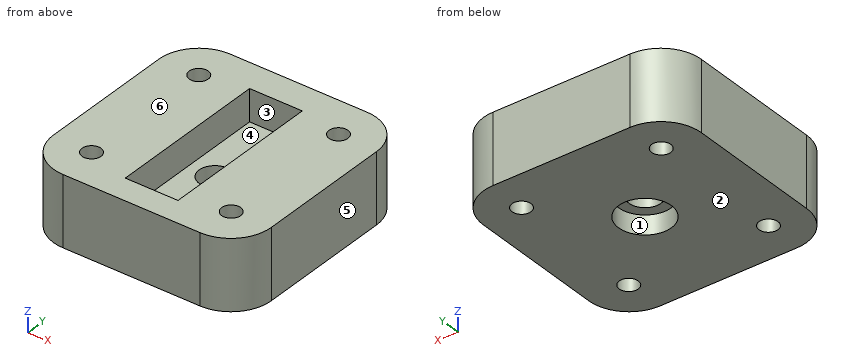
```python
from build123d import *

# Parameters (mm, degrees)
SKETCH1_W           = 34.29
SKETCH1_H           = 34.29
SKETCH1_R           = 1.5
BOSS_EXTRUDE1_DEPTH = 11
SKETCH2_W           = 8.3
SKETCH2_H           = 25.5
CUT_EXTRUDE1_DEPTH  = 5
SKETCH3_R           = 2.5
CUT_EXTRUDE2_DEPTH  = 5
SKETCH5_R           = 4.15
CUT_EXTRUDE4_DEPTH  = 3
FILLET2_R           = 6.35


with BuildPart() as part:
    # Sketch1 → Boss-Extrude1 (new body)
    with BuildSketch(Plane.XY):
        Rectangle(SKETCH1_W, SKETCH1_H)
        with Locations((-11, 11)):
            Circle(SKETCH1_R, mode=Mode.SUBTRACT)
        with Locations((11, 11)):
            Circle(SKETCH1_R, mode=Mode.SUBTRACT)
        with Locations((-11, -11)):
            Circle(SKETCH1_R, mode=Mode.SUBTRACT)
        with Locations((11, -11)):
            Circle(SKETCH1_R, mode=Mode.SUBTRACT)
    extrude(amount=BOSS_EXTRUDE1_DEPTH)

    # Sketch2 → Cut-Extrude1 (cut)
    with BuildSketch(Plane.XY.offset(11)):
        with Locations((0.041, -0.304)):
            Rectangle(SKETCH2_W, SKETCH2_H)
    extrude(amount=-CUT_EXTRUDE1_DEPTH, mode=Mode.SUBTRACT)

    # Sketch3 → Cut-Extrude2 (cut)
    with BuildSketch(Plane.XY.offset(6)):
        Circle(SKETCH3_R)
    extrude(amount=-CUT_EXTRUDE2_DEPTH, mode=Mode.SUBTRACT)

    # Sketch5 → Cut-Extrude4 (cut)
    with BuildSketch(Plane(origin=(0, 0, 0), x_dir=(-1, 0, 0), z_dir=(0, 0, -1))):
        Circle(SKETCH5_R)
    extrude(amount=-CUT_EXTRUDE4_DEPTH, mode=Mode.SUBTRACT)

    # Fillet2
    fillet2_edges = [part.edges().sort_by_distance(p)[0] for p in [
        (17.145, -17.145, 5.5),
        (-17.145, -17.145, 5.5),
        (-17.145, 17.145, 5.5),
        (17.145, 17.145, 5.5),
    ]]
    fillet(fillet2_edges, radius=FILLET2_R)


solid = part.part
```
Here's how the part is built. I have some questions about the finished solid (model axes, mm). Face numbers are marked on the shaded views. A direction names the side the tool comes from. Give positions to 0.01 mm unless a question says otherwise; leave off trailing zeros. Loops run counter-clockwise (first coordinate to the right, second up) from the corner with the lowest first, then second, coordinate; pieces in that order, holes last. Notation, with made-up numbers: M 78.25,33 L 94.25,33 A22 cw 94.25,50 Z; hole C 67,13.5 d9. An arc over 180 degrees is marked long. Return JSON: item names as keys, results as strings.
Item 1: Imagine slicing it at A-A on z = 7. List the corners of the cut face in (x, y) for me (3 decimals), then the cut area to 3 significant figures.
A:
{"outline": "M -17.145,-10.795 A6.35 ccw -10.795,-17.145 L 10.795,-17.145 A6.35 ccw 17.145,-10.795 L 17.145,10.795 A6.35 ccw 10.795,17.145 L -10.795,17.145 A6.35 ccw -17.145,10.795 Z; hole C -11,-11 d3; hole C -11,11 d3; hole M -4.109,-13.054 L 4.191,-13.054 L 4.191,12.446 L -4.109,12.446 Z; hole C 11,-11 d3; hole C 11,11 d3", "area": "901 mm^2"}
Item 2: Thinking about a two-plate mould opening in X: for the marked faces 4, 5 and 6, which applies, released by +X, released by -X, zero draft, split by the parting line, or undercut?
A:
{"face 4": "undercut", "face 5": "released by +X", "face 6": "zero draft"}
Item 3: On a 3-axis mill with a long thin cutter (end or side, diameter ignored), from which of +Z, -Z, +X, -X, +Y, -Y can I reach the whole of each face in a straight line? I mean the marked faces 1, 2 and 3. Say none if no direction works.
A:
{"face 1": "-Z", "face 2": "-Z, +X, -X, +Y, -Y", "face 3": "+Z"}
Item 4: I'm going to push flat-ended pins straight in: pin 1 Ø6.5 at (x, y) = (0, 0) entering from -Z; pin 2 Ø6.5 at (x, y) = (-1.5, 5.5) entering from +Z; pin 3 Ø1.5 at (x, y) = (-2.5, 7.5) entering from +Z; pin 4 Ø1 at (y, z) = (13, 8.5) entering from -X. Where does each tip first touch, or does it pass through?
A:
{"pin 1": "stops at z = 3", "pin 2": "stops at z = 11", "pin 3": "stops at z = 6", "pin 4": "stops at x = -16.91"}
Item 5: Imagine slicing it at D-D on z = 5. List the corners of the cut face in (x, y) for me (3 decimals), then the cut area to 3 significant figures.
A:
{"outline": "M -17.145,-10.795 A6.35 ccw -10.795,-17.145 L 10.795,-17.145 A6.35 ccw 17.145,-10.795 L 17.145,10.795 A6.35 ccw 10.795,17.145 L -10.795,17.145 A6.35 ccw -17.145,10.795 Z; hole C -11,-11 d3; hole C -11,11 d3; hole C 0,0 d5; hole C 11,-11 d3; hole C 11,11 d3", "area": "1,090 mm^2"}
Item 6: Imagine slicing it at C-C on y = -8.5. List the corners of the cut face in (x, z) for me (3 decimals), then the cut area to 3 significant figures.
A:
{"outline": "M -17.145,0 L 17.145,0 L 17.145,11 L 4.191,11 L 4.191,6 L -4.109,6 L -4.109,11 L -17.145,11 Z", "area": "336 mm^2"}
Item 7: Please list where these lines run through material, in increasing order: line 1 (Y direction, x = 11, z = 5); line 2 (Y direction, x = 0, z = 4.55) (3 decimals); line 3 (X direction, y = -11.5, z = 4.5).
A:
{"line 1": "y = -17.14 to -12.5, -9.5 to 9.5, 12.5 to 17.14", "line 2": "y = -17.145 to -2.5, 2.5 to 17.145", "line 3": "x = -17.11 to -12.41, -9.59 to 9.59, 12.41 to 17.11"}
Item 8: Imagine slicing it at B-B on y = 0. List the corners of the cut face in (x, z) for me (3 decimals), then the cut area to 3 significant figures.
A:
{"outline": "M -17.145,0 L -4.15,0 L -4.15,3 L -2.5,3 L -2.5,6 L -4.109,6 L -4.109,11 L -17.145,11 Z; M 2.5,3 L 4.15,3 L 4.15,0 L 17.145,0 L 17.145,11 L 4.191,11 L 4.191,6 L 2.5,6 Z", "area": "296 mm^2"}
